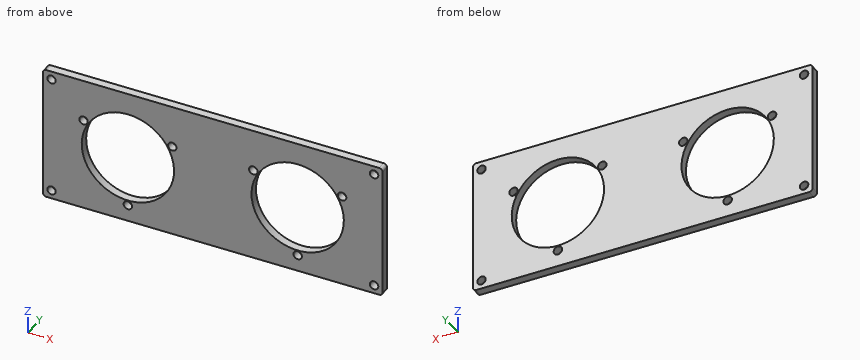
```python
from build123d import *

# Parameters (mm, degrees)
SKETCH1_W            = 127
SKETCH1_H            = 101.6
SKETCH1_R            = 34.544
SKETCH1_R_2          = 3.175
BOSS_EXTRUDE1_DEPTH  = 6.35
FILLET1_R            = 2.54
FILLET1_OF_MIRROR1_R = 2.54


with BuildPart() as part:
    # Sketch1 → Boss-Extrude1 (new body)
    with BuildSketch(Plane(origin=(0, 0, 0), x_dir=(1, 0, 0), z_dir=(0, 1, 0))):
        with Locations((63.5, 50.8)):
            Rectangle(SKETCH1_W, SKETCH1_H)
        with Locations(Location((63.5, 50.8, 0), (0, 0, 270))):
            Circle(SKETCH1_R, mode=Mode.SUBTRACT)
        with Locations(Location((6.35, 95.25, 0), (0, 0, 270))):
            Circle(SKETCH1_R_2, mode=Mode.SUBTRACT)
        with Locations(Location((6.35, 6.35, 0), (0, 0, 270))):
            Circle(SKETCH1_R_2, mode=Mode.SUBTRACT)
        with Locations(Location((63.5, 89.154, 0), (0, 0, 270))):
            Circle(SKETCH1_R_2, mode=Mode.SUBTRACT)
        with Locations(Location((96.715538337, 31.623, 0), (0, 0, 270))):
            Circle(SKETCH1_R_2, mode=Mode.SUBTRACT)
        with Locations(Location((30.284461663, 31.623, 0), (0, 0, 270))):
            Circle(SKETCH1_R_2, mode=Mode.SUBTRACT)
    boss_extrude1 = extrude(amount=BOSS_EXTRUDE1_DEPTH)

    # Fillet1
    fillet1_edges = [part.edges().sort_by_distance(p)[0] for p in [
        (0, 3.175, -101.6),
        (0, 3.175, 0),
    ]]
    fillet(fillet1_edges, radius=FILLET1_R)

    # Mirror1: Boss-Extrude1 across plane
    add(boss_extrude1.mirror(Plane(origin=(127, 6.35, 0), x_dir=(0, 0, 1), z_dir=(-1, 0, 0))))

    # Fillet1 of Mirror1
    fillet1_of_mirror1_edges = [part.edges().sort_by_distance(p)[0] for p in [
        (254, 3.175, -101.6),
        (254, 3.175, 0),
    ]]
    fillet(fillet1_of_mirror1_edges, radius=FILLET1_OF_MIRROR1_R)


solid = part.part
```
Input: part model. Units: mm. Frame: model coordinates. Round coordinates to 2 decimals unless told otherwise and drop trailing zeros. Order: outer loops, then holes, each group sorted by start corner. A loop starts at its lowest first (then second) coordinate and runs counter-clockwise, first axis right, second up. Notation, with made-up numbers: (16.5, -3.75) - (39.5, -3.75) arc R25 cw to (39.5, 19.25) - close; hole circle Ø11 at (89, 43.25). An arc over 180 degrees is marked (long way). Answer in a Markdown table with one row per item.
Item 1: Section query A-A (z = -50.8). Return the cut outline in (x, y).
Model answer:
| item | result |
|---|---|
| outline | (0, 0) - (28.96, 0) - (28.96, 6.35) - (0, 6.35) - close; (98.04, 0) - (155.96, 0) - (155.96, 6.35) - (98.04, 6.35) - close; (225.04, 0) - (254, 0) - (254, 6.35) - (225.04, 6.35) - close |
Item 2: Section query C-C (x = 84.5). Return the cut outline in (y, z).
Model answer:
| item | result |
|---|---|
| outline | (0, -101.6) - (6.35, -101.6) - (6.35, -78.23) - (0, -78.23) - close; (0, -23.37) - (6.35, -23.37) - (6.35, 0) - (0, 0) - close |
Item 3: Line query: line 1 (Z direction, x = 247.65, y = 5) (3 decimals); line 2 (Z direction, x = 190.5, y = 4.5); line 3 (X direction, y = 3.5, z = -50.8). Output: solid intervals per line, ascending.
Model answer:
| item | result |
|---|---|
| line 1 | z = -101.6 to -98.425, -92.075 to -9.525, -3.175 to 0 |
| line 2 | z = -101.6 to -92.33, -85.98 to -85.34, -16.26 to 0 |
| line 3 | x = 0 to 28.96, 98.04 to 155.96, 225.04 to 254 |
Item 4: Pin query (flat end, axial travel): pin 1 (4 mm diameter, centred on x = 96.72, z = -31.62, fed in from +Y). Return the tip coordinate at first contact, or that it passes through.
Model answer:
| item | result |
|---|---|
| pin 1 | passes through |
Item 5: Section query D-D (y = 1.25). Give the number of separate pieces and of enclosed holes in the cut face, then the cut area to 3 significant figures.
Model answer:
| item | result |
|---|---|
| separate pieces | 1 |
| enclosed holes | 12 |
| area | 18,000 mm² |
Item 6: Section query B-B (x = 247.65). Return the cut outline in (y, z) (3 decimals), then the cut area to 3 significant figures.
Model answer:
| item | result |
|---|---|
| outline | (0, -101.6) - (6.35, -101.6) - (6.35, -98.425) - (0, -98.425) - close; (0, -92.075) - (6.35, -92.075) - (6.35, -9.525) - (0, -9.525) - close; (0, -3.175) - (6.35, -3.175) - (6.35, 0) - (0, 0) - close |
| area | 565 mm² |
